Can you work these out from the model? Positions are in its coordinate system, mm. A direction names the side the tool comes from. Round coordinates to 2 decimals unless told otherwise and drop trailing zeros. Write each loop counter-clockwise with the first axis right and the second up, starting at its lowest first coordinate (ties: lowest second). Pieces come first, ordered by that corner, then holes. Notation, with made-up numbers: M 27,-32 L 71,-32 A19 ccw 71,-19 Z; hole C 31,48 d6. An arc over 180 degrees is marked long. Use one line per item in the form item = value. Start each with the question number.
```python
from build123d import *

# Parameters (mm, degrees)
SKETCH1_R                          = 10
BOSS_EXTRUDE1_DEPTH                = 15.5
F_2_0_2_DIAMETER_HOLE1_D           = 2
F_2_0_2_DIAMETER_HOLE1_DEPTH       = 2
F_2_0_2_DIAMETER_HOLE1_CSINK_D     = 2.05
F_2_0_2_DIAMETER_HOLE1_CSINK_ANGLE = 90
F_2_0_2_DIAMETER_HOLE1_TIP         = 0.600860619


with BuildPart() as part:
    # Sketch1 → Boss-Extrude1 (new body)
    with BuildSketch(Plane.XY):
        with BuildLine():
            Line((-10.84, -14.991477579), (10.84, -14.991477579))
            ThreePointArc((10.84, -14.991477579), (0, 18.5), (-10.84, -14.991477579))
        make_face()
        Circle(SKETCH1_R, mode=Mode.SUBTRACT)
    extrude(amount=BOSS_EXTRUDE1_DEPTH)

    # Ø2.0 (2) Diameter Hole1
    with Locations(Plane(origin=(0, -14.991477579, 0), x_dir=(-1, 0, 0), z_dir=(0, -1, 0))):
        with Locations((0, -7.75)):
            CounterSinkHole(F_2_0_2_DIAMETER_HOLE1_D / 2, F_2_0_2_DIAMETER_HOLE1_CSINK_D / 2, depth=F_2_0_2_DIAMETER_HOLE1_DEPTH, counter_sink_angle=F_2_0_2_DIAMETER_HOLE1_CSINK_ANGLE)
            with Locations((0, 0, -(F_2_0_2_DIAMETER_HOLE1_DEPTH + F_2_0_2_DIAMETER_HOLE1_TIP / 2))):  # 118° drill point
                Cone(0, F_2_0_2_DIAMETER_HOLE1_D / 2, F_2_0_2_DIAMETER_HOLE1_TIP, mode=Mode.SUBTRACT)


solid = part.part
```
1. Which directions (+Z, -Z, +X, -X, +Y, -Y) give clear straight access to the entire face, cutting with the end or side of a thin tool? Please do faces 4 (the face through (-4.4, 9.4, 0)), 5 (the face through (-0.13, -13.97, 6.76)).
2. Please list where these lines run through material, in increasing order: line 1 along Z through (x, y) = (0, -14.2); line 2 along Y through (x, z) = (-3.5, 1.25); line 3 along X through (y, z) = (6, 12.5).
3. If we section it at B-B (x = 2): List the corners of the cut face in (y, z) for me.
4. If we section it at A-A (y = 0): List the corners of the cut face in (x, z) for me.
5. Will these pins go through, and if not, where does the flat tip stop? pin 1 (4 mm diameter, centred on x = 9, z = 14, fed in from +Y); pin 2 (8 mm diameter, centred on y = -10, z = 5.5, fed in from -X).
6. If we section it at D-D (y = -11): List the corners of the cut face in (x, z) for me.
7. If we mould it in two halves opening along X, with no side actions, what happens to faces 1 (the face through (-2.17, -9.76, 7.64)), 2 (the face through (-4.4, 9.4, 15.5)), 3 (the face through (0.65, 18.49, 7.64))? For each: pulls with the +X half, pulls with the -X half, needs draft (parallel to the pull), parting line crosses it, or undercut.
8. If we section it at C-C (z = 4): List the corners of the cut face in (x, y) for me, and give its area (3 significant figures).
Model answer:
q1.face_4 = -Z, +X, -X, +Y, -Y
q1.face_5 = -Y
q2.line_1 = 0 to 6.75, 8.75 to 15.5
q2.line_2 = -14.99 to -9.37, 9.37 to 18.17
q2.line_3 = -17.5 to -8, 8 to 17.5
q3.outline = M -14.99,0 L -9.8,0 L -9.8,15.5 L -14.99,15.5 Z; M 9.8,0 L 18.39,0 L 18.39,15.5 L 9.8,15.5 Z
q4.outline = M -18.5,0 L -10,0 L -10,15.5 L -18.5,15.5 Z; M 10,0 L 18.5,0 L 18.5,15.5 L 10,15.5 Z
q5.pin_1 = 17.12
q5.pin_2 = -17.5
q6.outline = M -14.87,0 L 14.87,0 L 14.87,15.5 L -14.87,15.5 Z
q7.face_1 = undercut
q7.face_2 = needs draft
q7.face_3 = parting line crosses it
q8.outline = M -10.84,-14.99 L 10.84,-14.99 A18.5 ccw long Z; hole C 0,0 d20
q8.area = 709 mm2
